Source: CAD feature listing. Evaluate the final solid. Frame: model axes, mm. A direction names the side the tool comes from. Round coordinates to 2 decimals unless told otherwise and drop trailing zeros. Loops run counter-clockwise (first coordinate to the right, second up) from the corner with the lowest first, then second, coordinate; pieces in that order, holes last. Notation, with made-up numbers: (-14.5, -14) - (12.5, -14) arc R11 ccw to (12.5, -10) - close; hole circle Ø8 at (61, 48.5). An arc over 180 degrees is marked (long way). One line per question, with ' | ' between items.
from build123d import *

# Parameters (mm, degrees)
F0_R     = 3.175
F0_R_2   = 3.9751
F1_DEPTH = 3.175


with BuildPart() as f1:
    # F0 (on Front) → F1 (new body)
    with BuildSketch(Plane.XZ):
        with BuildLine():
            ThreePointArc((-12.7762, 44.45), (-20.6502, 52.324), (-28.5242, 44.45))
            Line((-28.5242, 44.45), (-31.8262, 0))
            ThreePointArc((-31.8262, 0), (-28.552825, -7.902625), (-20.6502, -11.176))
            Line((-20.6502, -11.176), (42.8498, -15.748))
            ThreePointArc((42.8498, -15.748), (58.5978, 0), (42.8498, 15.748))
            Line((42.8498, 15.748), (-3.109162, 12.438955))
            ThreePointArc((-3.109162, 12.438955), (-8.676921, 14.745196), (-10.983162, 20.312955))
            Line((-10.983162, 20.312955), (-12.7762, 44.45))
        make_face()
        with Locations((-20.6502, 0)):
            Circle(F0_R, mode=Mode.SUBTRACT)
        Circle(F0_R, mode=Mode.SUBTRACT)
        with Locations((42.8498, 0)):
            Circle(F0_R_2, mode=Mode.SUBTRACT)
        with Locations((-20.6502, 44.45)):
            Circle(F0_R, mode=Mode.SUBTRACT)
    extrude(amount=F1_DEPTH)


solid = f1.part
1. Section query D-D, the plane z = 37. Return loops of the section in (x, y) (3 decimals), plus the area to 3 significant figures.
Worked out:
outline: (-29.078, -3.175) - (-12.223, -3.175) - (-12.223, 0) - (-29.078, 0) - close | area: 53.5 mm2
2. Material intervals for probe 1 along X at (y, z) = (-2.7, 11.5); probe 2 along Z at (x, y) = (-14, -0.1); probe 3 along Z at (x, y) = (25.5, -2.4), sorted ascending.
Worked out:
probe 1: x = -30.97 to 53.61 | probe 2: z = -11.65 to 48.67 | probe 3: z = -14.5 to 14.5
3. Section query C-C, the plane x = 26.5. Return loops of the section in (y, z) (3 decimals), plus the area to 3 significant figures.
Worked out:
outline: (-3.175, -14.571) - (0, -14.571) - (0, 14.571) - (-3.175, 14.571) - close | area: 92.5 mm2
4. Access query for faces 4 (the cylindrical face through (-8.615, -1.565, 14.684)), 5 (the cylindrical face through (-23.822, -1.565, 0.14)). Directions: +Z, -Z, +X, -X, +Y, -Y. A direction counts if a zero-diameter tool reaches every point of the face in a straight line with its end or side. Return the directions, or none.
Worked out:
face 4: +Z, +Y, -Y | face 5: +Y, -Y
5. Section query B-B, the plane x = 0. Return loops of the section in (y, z) (3 decimals).
Worked out:
outline: (-3.175, -12.663) - (0, -12.663) - (0, -3.175) - (-3.175, -3.175) - close; (-3.175, 3.175) - (0, 3.175) - (0, 12.663) - (-3.175, 12.663) - close
6. Contact query for flat-ended pins moving along their axis: P1, Ø8.5, axis at x = -20.65, z = 0, coming from the +Y side; P2, Ø5.5, axis at x = 0, z = 0, coming from the +Y side; P3, Ø1.5, axis at y = -1, z = 40, coming from the +X side. Output: stop coordinate, or through.
Worked out:
P1: stops at y = 0 | P2: passes through | P3: stops at x = -12.39
7. Section query A-A, the plane y = -1.85. Return loops of the section in (x, z) (3 decimals), plus the area to 3 significant figures.
Worked out:
outline: (-31.826, 0) arc R11.176 ccw to (-20.65, -11.176) - (42.85, -15.748) arc R15.748 ccw to (42.85, 15.748) - (-3.109, 12.439) arc R7.874 cw to (-10.983, 20.313) - (-12.776, 44.45) arc R7.874 ccw to (-28.524, 44.45) - close; hole circle Ø6.35 at (-20.65, 0); hole circle Ø6.35 at (-20.65, 44.45); hole circle Ø6.35 at (0, 0); hole circle Ø7.95 at (42.85, 0) | area: 2,890 mm2
8. Mould query, pull axis Z, two halves, no side actions, for faces 1 (the flat face through (10.66, -1.57, -13.43)), 2 (the cylindrical face through (46.641, -1.565, 1.194)), 3 (the flat face through (20.192, -1.565, 14.117)). Classes: released by +Z, released by -Z, zero draft, split by the parting line, or undercut.
Worked out:
face 1: released by -Z | face 2: undercut | face 3: released by +Z
